Verification items for this drawing (mm, ordinates from the low corner). Coordinates: 2 decimals unless noted, no trailing zeros. Write each loop counter-clockwise with the first axis right and the second up, starting at its lowest first coordinate (ties: lowest second). Pieces come first, ordered by that corner, then holes. Notation, with made-up numbers: M 9,-5 L 41,-5 A35 cw 41,34 Z; hole C -25.5,4.5 d6. An arc over 180 degrees is marked long. Answer as CSV lines item,"result". Start each with the question number.
1) Section check B-B (x = 34.5). Record the cut outline in (y, z).
2) Material ranges on L1, parallel to X at y = 2.8, z = 37.5 (3 decimals); L2, parallel to X at y = 2.9, z = 44; L3, parallel to X at y = 2.8, z = 81.5 (3 decimals), recorded low to high. Write a range as [from, to].
3) Section check C-C (z = 23.5). Record the cut outline in (x, y) (3 decimals), and give its area (3 significant figures).
4) Go/stop test with flat-tipped pins: pin 1 Ø1 at (y, z) = (2, 76.5) entering from -X (3 decimals); pin 2 Ø2 at (y, z) = (1.5, 31) entering from +X (3 decimals); pin 3 Ø1 at (x, y) = (1.5, 2.5) entering from +Z. Record where each tip stops, or that it passes through.
5) Section check A-A (y = 2.25). Record the cut outline in (x, z) (3 decimals), and give its area (3 significant figures).
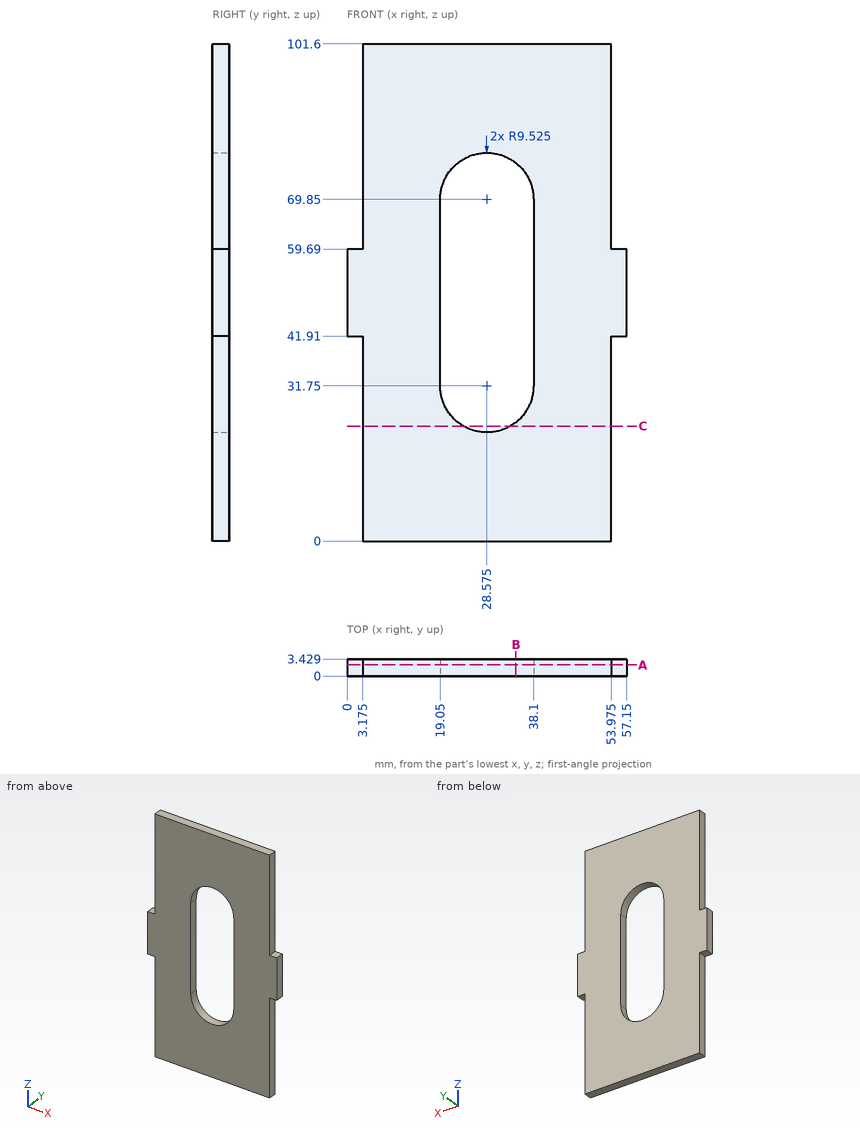
Results found:
1,outline,"M 0,0 L 3.43,0 L 3.43,24.29 L 0,24.29 Z; M 0,77.31 L 3.43,77.31 L 3.43,101.6 L 0,101.6 Z"
2,L1,"x = [3.175, 19.05], [38.1, 53.975]"
2,L2,"x = [0, 19.05], [38.1, 57.15]"
2,L3,"x = [3.175, 53.975]"
3,outline,"M 3.175,0 L 23.814,0 L 23.814,3.429 L 3.175,3.429 Z; M 33.336,0 L 53.975,0 L 53.975,3.429 L 33.336,3.429 Z"
3,area,"142 mm2"
4,pin 1,"stops at x = 3.175"
4,pin 2,"stops at x = 53.975"
4,pin 3,"stops at z = 59.69"
5,outline,"M 0,41.91 L 3.175,41.91 L 3.175,0 L 53.975,0 L 53.975,41.91 L 57.15,41.91 L 57.15,59.69 L 53.975,59.69 L 53.975,101.6 L 3.175,101.6 L 3.175,59.69 L 0,59.69 Z; hole M 19.05,31.75 A9.525 ccw 38.1,31.75 L 38.1,69.85 A9.525 ccw 19.05,69.85 Z"
5,area,"4,260 mm2"
